Check sheet for the modelled part. Datum: model origin and axes. Units: mm. Face numbers are marked on the shaded views. Coordinates: 2 decimals unless noted, no trailing zeros. Write each loop counter-clockwise with the first axis right and the second up, starting at its lowest first coordinate (ties: lowest second). Pieces come first, ordered by that corner, then holes. Notation, with made-up numbers: (27, 27) -> (52, 27) arc R35 cw to (52, 63) -> close; hole circle Ø8 at (-18.75, -6). An arc over 180 degrees is marked (long way). Put each result on its own line as item: value.
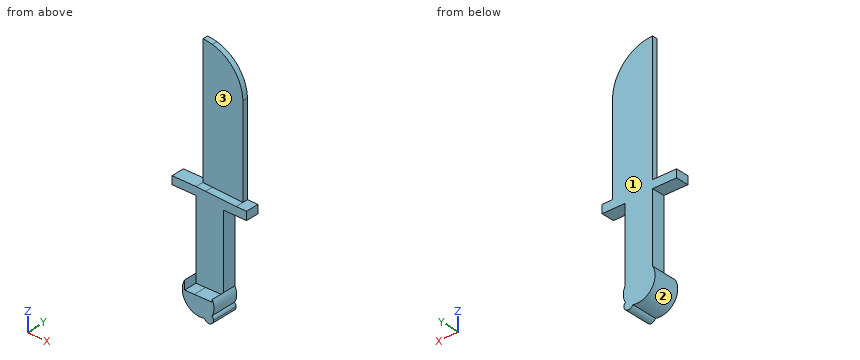
```python
from build123d import *

# Parameters (mm, degrees)
F1_DEPTH = 5.08
F2_DEPTH = 12.7
F3_DEPTH = 25.4


with BuildPart() as f1:
    # F0 (on Front) → F1 (new body)
    with BuildSketch(Plane.XZ):
        with BuildLine():
            Line((0, -47.187425), (0, 75.595615))
            ThreePointArc((0, 75.595615), (-4.619314, 76.443648), (-9.307228, 76.727711))
            Line((-9.307228, 76.727711), (-9.307228, 37.903182))
            Line((-9.307228, 37.903182), (-9.307228, -46.803496))
            Line((-9.307228, -46.803496), (0, -47.187425))
        make_face()
        with BuildLine():
            ThreePointArc((29.501495, 39.010878), (20.91523, 62.274211), (0, 75.595615))
            Line((0, 75.595615), (0, -47.187425))
            Line((0, -47.187425), (29.501495, -48.404383))
            Line((29.501495, -48.404383), (29.501495, -27.950756))
            Line((29.501495, -27.950756), (29.501495, 0))
            Line((29.501495, 0), (29.501495, 39.010878))
        make_face()
    extrude(amount=F1_DEPTH)

    # F0 (on Front) → F2 (join)
    with BuildSketch(Plane.XZ):
        Polygon((29.501495, -48.404383), (0, -47.187425), (-9.307228, -46.803496), (-32.457575, -46.803496), (-32.457575, -54.546013), (-9.307228, -54.546013), (-9.307228, -121.184757), (-9.307228, -129.937008), (0, -129.937008), (17.238326, -129.725629), (17.238326, -127.477206), (17.238326, -79.020567), (17.238326, -56.486391), (29.501495, -56.486391), (39.612059, -56.486391), (39.612059, -48.404383), align=None)
    extrude(amount=F2_DEPTH)

    # F0 (on Front) → F3 (join)
    with BuildSketch(Plane.XZ):
        with BuildLine():
            Line((-9.307228, -129.937008), (-9.307228, -121.184757))
            ThreePointArc((-9.307228, -121.184757), (-8.169823, -140.263142), (9.859656, -146.604776))
            ThreePointArc((9.859656, -146.604776), (11.990386, -145.914729), (14.013868, -144.954681))
            ThreePointArc((14.013868, -144.954681), (15.649123, -143.419867), (17.007979, -141.635709))
            ThreePointArc((17.007979, -141.635709), (19.126457, -134.58905), (17.238326, -127.477206))
            Line((17.238326, -127.477206), (17.238326, -129.725629))
            Line((17.238326, -129.725629), (0, -129.937008))
            Line((0, -129.937008), (-9.307228, -129.937008))
        make_face()
        with BuildLine():
            ThreePointArc((14.013868, -144.954681), (11.990386, -145.914729), (9.859656, -146.604776))
            ThreePointArc((9.859656, -146.604776), (14.853881, -149.344973), (18.483799, -144.954681))
            ThreePointArc((18.483799, -144.954681), (18.098213, -143.13853), (17.007979, -141.635709))
            ThreePointArc((17.007979, -141.635709), (15.649123, -143.419867), (14.013868, -144.954681))
        make_face()
    extrude(amount=F3_DEPTH)


solid = f1.part
```
Q1. Mould release check, pull along Y, two halves, no side actions. Record for the marked faces 1, 2 and 3: released by +Y, released by -Y, zero draft, split by the parting line, or undercut.
Recorded:
face 1: released by +Y
face 2: zero draft
face 3: released by -Y
Q2. Material ranges on line 1 along Y through (x, z) = (15, 46); line 2 along Z through (x, y) = (-10, -2); line 3 along Z through (x, y) = (32, -9.5), recorded low to high.
Recorded:
line 1: y = -5.08 to 0
line 2: z = -137.23 to -122.5, -54.55 to -46.8
line 3: z = -56.49 to -48.4
Q3. Cross-section at D-D (z = 0.5). Record the cut outline in (x, y).
Recorded:
outline: (-9.31, -5.08) -> (29.5, -5.08) -> (29.5, 0) -> (-9.31, 0) -> close
Q4. Cross-section at B-B (y = -16.25). Record the cut outline in (x, z), plus the area to 3 significant figures.
Recorded:
outline: (-9.31, -129.94) -> (-9.31, -121.18) arc R17.27 ccw to (9.86, -146.6) arc R4.47 ccw to (18.48, -144.95) arc R4.47 ccw to (17.01, -141.64) arc R13.51 ccw to (17.24, -127.48) -> (17.24, -129.73) -> (0, -129.94) -> close
area: 483 mm2
Q5. Cross-section at A-A (x = 22.5). Record the cut outline in (y, z), plus the area to 3 significant figures.
Recorded:
outline: (-12.7, -56.49) -> (0, -56.49) -> (0, 60.17) -> (-5.08, 60.17) -> (-5.08, -48.12) -> (-12.7, -48.12) -> close
area: 656 mm2
Q6. Depth check by flat-ended pin: P1, Ø2.5, axis at y = -18, z = -129, coming from the -X side; P2, Ø1.5, axis at y = -3.5, z = 10, coming from the +X side; P3, Ø5.5, axis at y = -3, z = -11.5, coming from the -X side; P4, Ø3, axis at y = -7.5, z = 25.5, coming from the +X side. Enter the tip coordinate at first touch or a pass-through.
Recorded:
P1: stops at x = -11.65
P2: stops at x = 29.5
P3: stops at x = -9.31
P4: passes through
Q7. Cross-section at C-C (z = -69). Record the cut outline in (x, y).
Recorded:
outline: (-9.31, -12.7) -> (17.24, -12.7) -> (17.24, 0) -> (-9.31, 0) -> close
